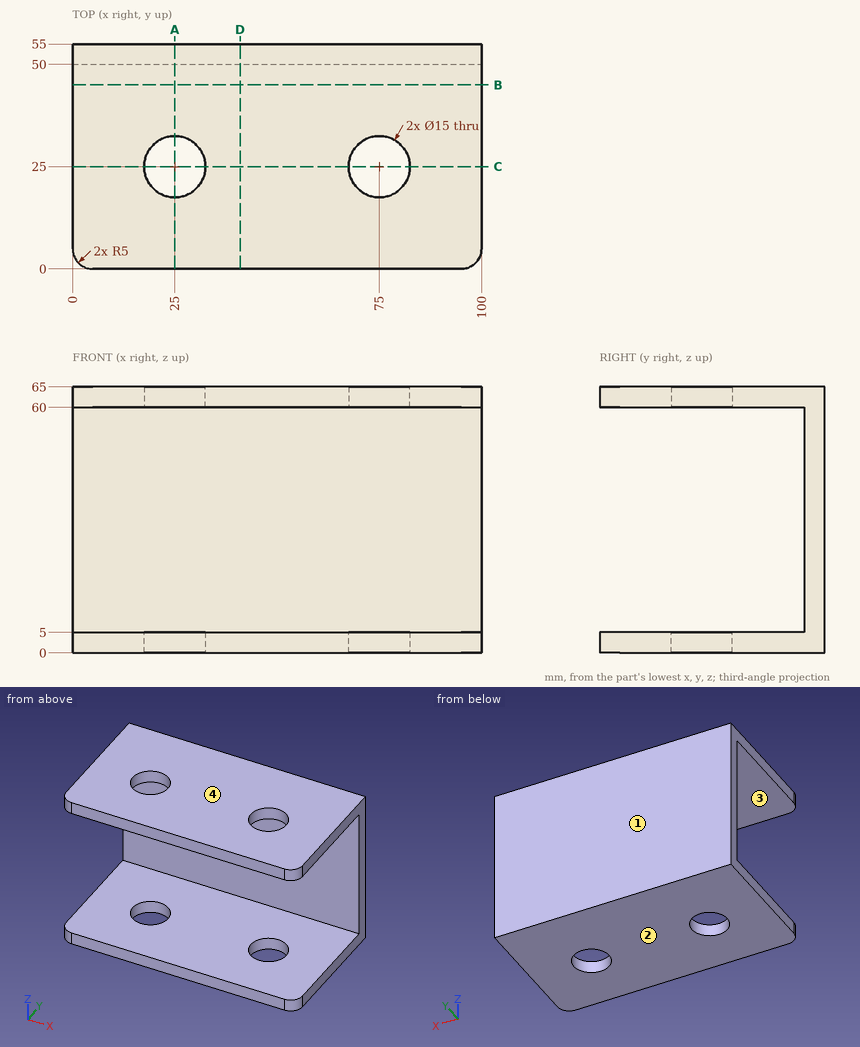
Answer from the drawing. Dimensions are ordinates in mm from the lowest x, y and z of the part. Round coordinates to 2 decimals unless told otherwise and drop trailing zeros. Loops run counter-clockwise (first coordinate to the right, second up) from the corner with the lowest first, then second, coordinate; pieces in that order, holes last.
1) Consider line 1 (X direction, y = 25.5, z = 3); line 2 (Z direction, x = 69, y = 42.5); line 3 (Y direction, x = 75, z = 1.45). Determine where each line is inside the solid, lowest interval first.
Outcome:
line 1: x = 0 to 17.52, 32.48 to 67.52, 82.48 to 100
line 2: z = 0 to 5, 60 to 65
line 3: y = 0 to 17.5, 32.5 to 55
2) A cutting plane is placed at A-A on x = 25. Determine the outline of the cut face in (y, z), plus the area to 3 significant figures.
Outcome:
outline: (0, 0) - (17.5, 0) - (17.5, 5) - (0, 5) - close; (0, 60) - (17.5, 60) - (17.5, 65) - (0, 65) - close; (32.5, 0) - (55, 0) - (55, 65) - (32.5, 65) - (32.5, 60) - (50, 60) - (50, 5) - (32.5, 5) - close
area: 675 mm2
3) A cutting plane is placed at B-B on y = 45. Determine the outline of the cut face in (x, z).
Outcome:
outline: (0, 0) - (100, 0) - (100, 5) - (0, 5) - close; (0, 60) - (100, 60) - (100, 65) - (0, 65) - close
4) A cutting plane is placed at C-C on y = 25. Determine the outline of the cut face in (x, z).
Outcome:
outline: (0, 0) - (17.5, 0) - (17.5, 5) - (0, 5) - close; (0, 60) - (17.5, 60) - (17.5, 65) - (0, 65) - close; (32.5, 0) - (67.5, 0) - (67.5, 5) - (32.5, 5) - close; (32.5, 60) - (67.5, 60) - (67.5, 65) - (32.5, 65) - close; (82.5, 0) - (100, 0) - (100, 5) - (82.5, 5) - close; (82.5, 60) - (100, 60) - (100, 65) - (82.5, 65) - close
5) Given P1, Ø12, axis at y = 25, z = 52.5, coming from the -X side; P2, Ø12, axis at x = 46, z = 41, coming from the -Y side; P3, Ø24, axis at x = 75, y = 25, coming from the -Z side, each flat-ended and moving along its own axis, determine where each tip first touches the part or whether it passes through.
Outcome:
P1: passes through
P2: stops at y = 50
P3: stops at z = 0
6) A cutting plane is placed at D-D on x = 41. Determine the outline of the cut face in (y, z).
Outcome:
outline: (0, 0) - (55, 0) - (55, 65) - (0, 65) - (0, 60) - (50, 60) - (50, 5) - (0, 5) - close
7) For a pull along Z with two mould halves and no side action, classify the marked faces 1, 2, 3 and 4 as released by +Z, released by -Z, zero draft, split by the parting line, or undercut.
Outcome:
face 1: zero draft
face 2: released by -Z
face 3: undercut
face 4: released by +Z
